```python
from build123d import *

# Parameters (mm, degrees)
F1_DEPTH = 50
F2_F1_R  = 5
F2_F2_R  = 5
F3_W     = 10
F3_H     = 10
F3_R     = 3
F4_DEPTH = 50
F5_R     = 4.99999
F6_W     = 30
F6_H     = 14.961473023
F7_DEPTH = 25


# Not quite as in the source:
# - a fillet or chamfer is up to 0.001 mm smaller than in the source, because OpenCascade refuses the exact size


with BuildPart() as f1:
    # F0 (on Right) → F1 (new body)
    with BuildSketch(Plane.YZ):
        Polygon((-95, 0), (0, 0), (0, 10), (-70, 10), (-70, 70), (-82.7777751063, 70), (-95, 70), (-95, 60), (-80, 60), (-80, 10), (-95, 10), align=None)
    extrude(amount=F1_DEPTH)

    # F2: fillet of radius 5 on 8 edges, made by hand

    # F2_f1
    f2_f1_edges = [f1.edges().sort_by_distance(p)[0] for p in [
        (25, -70, 10),
    ]]
    fillet(f2_f1_edges, radius=F2_F1_R)

    # F2_f2
    f2_f2_edges = [f1.edges().sort_by_distance(p)[0] for p in [
        (25, -70, 70),
        (50, -82.5, 70),
        (0, -82.5, 70),
        (25, 0, 10),
        (50, -32.5, 10),
        (0, -32.5, 10),
        (25, -95, 70),
        (0, -68.5355339059, 11.4644660941),
        (50, -68.5355339059, 11.4644660941),
    ]]
    fillet(f2_f2_edges, radius=F2_F2_R)

    # F3 (on face) → F4 (join)
    with BuildSketch(Plane.YZ.offset(50)):
        with Locations((-80, -5)):
            Rectangle(F3_W, F3_H)
        with Locations((-80, -5)):
            Circle(F3_R, mode=Mode.SUBTRACT)
        with Locations((-15, -5)):
            Rectangle(F3_W, F3_H)
        with Locations((-15, -5)):
            Circle(F3_R, mode=Mode.SUBTRACT)
    extrude(amount=-F4_DEPTH)

    # F5 (radius 5 in the source; OpenCascade refuses exactly that, so slightly less here)
    f5_edges = [f1.edges().sort_by_distance(p)[0] for p in [
        (25, -75, -10),
        (25, -85, -10),
        (25, -20, -10),
        (25, -10, -10),
    ]]
    fillet(f5_edges, radius=F5_R)

    # F6 (on face) → F7 (cut)
    with BuildSketch(Plane(origin=(0, -70, 0), x_dir=(-1, 0, 0), z_dir=(0, 1, 0))):
        with Locations((-25, 57.5192634885)):
            Rectangle(F6_W, F6_H)
    extrude(amount=-F7_DEPTH, mode=Mode.SUBTRACT)


solid = f1.part
```
Can you work these out from the model? Positions are in its coordinate system, mm. A direction names the side the tool comes from. Give positions to 0.01 mm unless a question says otherwise; leave off trailing zeros. Write each loop counter-clockwise with the first axis right and the second up, starting at its lowest first coordinate (ties: lowest second). Pieces come first, ordered by that corner, then holes. Notation, with made-up numbers: (-4, 1.25) - (9, 1.25) arc R20 cw to (9, 11.25) - close; hole circle Ø6 at (-38, -13.5). An arc over 180 degrees is marked (long way). Write item = value, one per line. Start each with the question number.
1. Imagine slicing it at D-D (y = -55). Please give me the cut outline in (x, z).
2. Please list where these lines run through material, in increasing order: line 1 (Y direction, x = 7.5, z = -0.5); line 2 (Z direction, x = 21.5, y = -15); line 3 (Z direction, x = 41, y = -87).
3. Thinking about a two-plate mould opening in X: for faces 1 (the face through (25, -87, 10)), 2 (the face through (48, -71, 40)), 3 (the face through (25, -82, 65)), 4 (the face through (1, -85, 68)), which applies, released by +X, released by -X, zero draft, split by the parting line, or undercut?
4. On a 3-axis mill with a long thin cutter (end or side, diameter ignored), from which of +Z, -Z, +X, -X, +Y, -Y can I reach the whole of each face in a straight line? I mean faces 5 (the face through (25, -90, 0)), 6 (the face through (25, -5, 0)), 7 (the face through (45, -88, 60)), 8 (the face through (25, -70, 34)), 9 (the face through (25, -20, -3)). Say none if no direction works.
5. For pin 1 (1.5 mm diameter, centred on x = 36, z = -3, fed in from +Y); pin 2 (2 mm diameter, centred on x = 18.5, y = -78, fed in from -Z); pin 3 (25 mm diameter, centred on x = 20.5, y = -47, fed in from -Z), each with a flat end and sliding along its axis, tell me the tip position at first contact or that it passes through.
6. Imagine slicing it at C-C (z = 18). Please give me the cut outline in (x, y), and give its area (3 significant figures).
7. Imagine slicing it at B-B (z = 53). Please give me the cut outline in (x, y), and give its area (3 significant figures).
8. Imagine slicing it at A-A (x = 13). Count the separate pieces of the cut face and the enclosed holes in it, and give its area (3 significant figures).
Worked answers:
q1.outline = (0, 0) - (50, 0) - (50, 5) arc R5 ccw to (45, 10) - (5, 10) arc R5 ccw to (0, 5) - close
q2.line_1 = -85 to -75, -20 to -10
q2.line_2 = -10 to -8, -2 to 10
q2.line_3 = 0 to 10, 60 to 70
q3.face_1 = zero draft
q3.face_2 = released by +X
q3.face_3 = undercut
q3.face_4 = released by -X
q4.face_5 = -Z, +X, -X, -Y
q4.face_6 = -Z, +X, -X, +Y
q4.face_7 = +X, -X, -Y
q4.face_8 = +Z, +X, -X, +Y
q4.face_9 = -Z, +X, -X
q5.pin_1 = -10
q5.pin_2 = -9.9
q5.pin_3 = 0
q6.outline = (0, -80) - (50, -80) - (50, -75) arc R5 ccw to (45, -70) - (5, -70) arc R5 ccw to (0, -75) - close
q6.area = 489 mm2
q7.outline = (0, -80) - (10, -80) - (10, -70) - (5, -70) arc R5 ccw to (0, -75) - close; (40, -80) - (50, -80) - (50, -75) arc R5 ccw to (45, -70) - (40, -70) - close
q7.area = 189 mm2
q8.separate_pieces = 2
q8.enclosed_holes = 2
q8.area = 1,590 mm2
